```python
from build123d import *

# Parameters (mm, degrees)
F0_W     = 28.575
F0_H     = 38.1
F1_DEPTH = 38.1
F3_DEPTH = 28.575
F4_D     = 12.7
F4_DEPTH = 12.7
F4_TIP   = 3.8154649308


with BuildPart() as f1:
    # F0 (on Top) → F1 (new body)
    with BuildSketch(Plane.XY):
        Rectangle(F0_W, F0_H)
    extrude(amount=F1_DEPTH)

    # F2 (on face) → F3 (join, through all)
    with BuildSketch(Plane.YZ.offset(14.2875)):
        with BuildLine():
            ThreePointArc((-19.05, 38.1), (-25.4, 19.05), (-19.05, 0))
            Line((-19.05, 0), (-19.05, 38.1))
        make_face()
        with BuildLine():
            Line((19.05, 38.1), (19.05, 0))
            ThreePointArc((19.05, 0), (25.4, 19.05), (19.05, 38.1))
        make_face()
    extrude(amount=-F3_DEPTH)

    # F4
    with Locations(Plane.YZ.offset(14.2875)):
        with Locations((-6.35, 19.05)):
            Hole(F4_D / 2, depth=F4_DEPTH)
            with Locations((0, 0, -(F4_DEPTH + F4_TIP / 2))):  # 118° drill point
                Cone(0, F4_D / 2, F4_TIP, mode=Mode.SUBTRACT)


solid = f1.part
```
Design review of the part built by this model. Coordinates are the model's own, in mm. Coordinates: 2 decimals unless noted, no trailing zeros. Order: outer loops, then holes, each group sorted by start corner. A loop starts at its lowest first (then second) coordinate and runs counter-clockwise, first axis right, second up. Notation, with made-up numbers: (69, 28.25) - (93, 28.25) arc R11 cw to (93, 38.25) - close; hole circle Ø1 at (39, 48.5). An arc over 180 degrees is marked (long way). Answer in a Markdown table with one row per item.
(1) The part is to be moulded in two halves that separate along Z. For faces 1 (the cylindrical face through (0.2, -25.4, 19.3)), 2 (the flat face through (0, 0, 38.1)), 3 (the cylindrical face through (7.849, -9.764, 24.404)), 4 (the conical face through (-1.565, -5.841, 18.072)), say which applies: released by +Z, released by -Z, zero draft, split by the parting line, or undercut.
Checked values:
| item | result |
|---|---|
| face 1 | split by the parting line |
| face 2 | released by +Z |
| face 3 | undercut |
| face 4 | undercut |
(2) Wall thickness on line 1 along Y through (x, z) = (5.5, 19.05); line 2 along Z through (x, y) = (11.5, -6.35); line 3 along Y through (x, z) = (-1, 30.5): over which ranges is each line inside the solid? List them lowest first. Write a range as from..to.
Checked values:
| item | result |
|---|---|
| line 1 | -25.4..-12.7, 0..25.4 |
| line 2 | 0..12.7, 25.4..38.1 |
| line 3 | -23.26..23.26 |
(3) Consider section D-D on y = 20.5. State the section outline as (x, z) points, plus the area to 3 significant figures.
Checked values:
| item | result |
|---|---|
| outline | (-14.29, 2.1) - (14.29, 2.1) - (14.29, 36) - (-14.29, 36) - close |
| area | 968 mm^2 |
(4) Consider section B-B on z = 26. State the section outline as (x, y) points.
Checked values:
| item | result |
|---|---|
| outline | (-14.29, -24.63) - (14.29, -24.63) - (14.29, 24.63) - (-14.29, 24.63) - close |
(5) Clearance check with flat-ended pins moving along their axes: pin 1 (10 mm diameter, centred on x = 7, z = 5, fed in from +Y); pin 2 (10 mm diameter, centred on x = 4, z = 15, fed in from -Y); pin 3 (1.5 mm diameter, centred on x = 2.5, z = 21, fed in from +Y). State where each tip first meets the part, or that it passes through.
Checked values:
| item | result |
|---|---|
| pin 1 | y = 24.08 |
| pin 2 | y = -25.4 |
| pin 3 | y = 25.38 |
(6) Consider section C-C on x = 1. State the section outline as (y, z) points, plus the area to 3 significant figures.
Checked values:
| item | result |
|---|---|
| outline | (-19.05, 0) - (19.05, 0) arc R31.75 ccw to (19.05, 38.1) - (-19.05, 38.1) arc R31.75 ccw to start; hole circle Ø10.74 at (-6.35, 19.05) |
| area | 1,690 mm^2 |
(7) Consider section A-A on x = 11.75. State the section outline as (y, z) points.
Checked values:
| item | result |
|---|---|
| outline | (-19.05, 0) - (19.05, 0) arc R31.75 ccw to (19.05, 38.1) - (-19.05, 38.1) arc R31.75 ccw to start; hole circle Ø12.7 at (-6.35, 19.05) |
